```python
from build123d import *

# Parameters (mm, degrees)
BOSS_EXTRUDE1_DEPTH = 150
BOSS_EXTRUDE2_DEPTH = 150


with BuildPart() as part:
    # Sketch1 → Boss-Extrude1 (new body)
    with BuildSketch(Plane.XY):
        with BuildLine():
            Line((32.688132281, -32.688132281), (35.382209117, -35.382209117))
            ThreePointArc((35.382209117, -35.382209117), (0, -50.038), (-35.382209117, -35.382209117))
            Line((-35.382209117, -35.382209117), (-32.688132281, -32.688132281))
            ThreePointArc((-32.688132281, -32.688132281), (0, -46.228), (32.688132281, -32.688132281))
        make_face()
    extrude(amount=-BOSS_EXTRUDE1_DEPTH)

    # Sketch2 → Boss-Extrude2 (add)
    with BuildSketch(Plane.XY):
        with BuildLine():
            Line((-9.525, -36.775), (-28.011200599, -36.775))
            ThreePointArc((-28.011200599, -36.775), (-14.781631913, -43.801042704), (0, -46.228))
            Line((0, -46.228), (0, -45.609510869))
            Line((0, -45.609510869), (-4.445, -45.609510869))
            Line((-4.445, -45.609510869), (-4.445, -44.085510869))
            Line((-4.445, -44.085510869), (-12.622621116, -44.085510869))
            ThreePointArc((-12.622621116, -44.085510869), (-13.192135307, -43.731364187), (-13.126400487, -43.063947362))
            Line((-13.126400487, -43.063947362), (-9.525, -38.370510869))
            Line((-9.525, -38.370510869), (-9.525, -36.775))
        make_face()
        with BuildLine():
            Line((0, -45.609510869), (0, -46.228))
            ThreePointArc((0, -46.228), (14.781631913, -43.801042704), (28.011200599, -36.775))
            Line((28.011200599, -36.775), (9.525, -36.775))
            Line((9.525, -36.775), (9.525, -38.370510869))
            Line((9.525, -38.370510869), (13.126400487, -43.063947362))
            ThreePointArc((13.126400487, -43.063947362), (13.192135307, -43.731364187), (12.622621116, -44.085510869))
            Line((12.622621116, -44.085510869), (4.445, -44.085510869))
            Line((4.445, -44.085510869), (4.445, -45.609510869))
            Line((4.445, -45.609510869), (0, -45.609510869))
        make_face()
    extrude(amount=-BOSS_EXTRUDE2_DEPTH)


solid = part.part
```
Can you work these out from the model? Positions are in its coordinate system, mm. A direction names the side the tool comes from. Give positions to 0.01 mm unless a question says otherwise; leave off trailing zeros. Loops run counter-clockwise (first coordinate to the right, second up) from the corner with the lowest first, then second, coordinate; pieces in that order, holes last. Notation, with made-up numbers: M -13.5,71 L 12.5,71 A23 ccw 12.5,92 Z; hole C 27.5,76.25 d3. An arc over 180 degrees is marked long. Use CSV: the item, a comma, the result in double quotes. Start each with the question number.
1. If I drill on L1, parallel to X at y = -36, z = -101.5; L2, parallel to Y at x = -1, z = -116; L3, parallel to X at y = -40.25, z = -141, over which ranges is the centre line in solid material (lowest first)?
2. For P1, Ø0.8, axis at y = -45, z = -83, coming from the -X side; P2, Ø5, axis at x = -15.5, z = -130.5, coming from the +Y side (3 decimals); P3, Ø0.8, axis at y = -45, z = -70, coming from the +X side; P4, Ø8, axis at x = -19.5, y = -45, coming from the +Z side, each with a flat end and sliding along its axis, tell me the tip position at first contact or that it passes through.
3. Imagine slicing it at A-A, the plane z = -44. Write out the boundary of the cut face in (x, y) (3 decimals), plus the area to 3 significant figures.
4. If we mould it in two halves opening along Y, with no side actions, what happens to faces 1 (the face through (0, -45.61, -74)), 2 (the face through (9, -44.086, -74)), 3 (the face through (0.55, -50.035, -73.95))? For each: released by +Y, released by -Y, zero draft, split by the parting line, or undercut.
5. On a 3-axis mill with a long thin cutter (end or side, diameter ignored), from which of +Z, -Z, +X, -X, +Y, -Y can I reach the whole of each face in a straight line? I mean faces 4 (the face through (-30.45, -34.78, -73.95)), 5 (the face through (-8, -44.086, -74)), 6 (the face through (34, -34, -74)). Say none if no direction works.
Response values:
1,L1,"-34.75 to -29, 29 to 34.75"
1,L2,"-50.03 to -45.61"
1,L3,"-29.73 to -10.97, 10.97 to 29.73"
2,P1,"x = -22.69"
2,P2,"y = -36.775"
2,P3,"x = 22.69"
2,P4,"z = 0"
3,outline,"M -35.382,-35.382 A50.038 ccw 35.382,-35.382 L 32.688,-32.688 A46.228 cw 28.011,-36.775 L 9.525,-36.775 L 9.525,-38.371 L 13.126,-43.064 A0.635 cw 12.623,-44.086 L 4.445,-44.086 L 4.445,-45.61 L -4.445,-45.61 L -4.445,-44.086 L -12.623,-44.086 A0.635 cw -13.126,-43.064 L -9.525,-38.371 L -9.525,-36.775 L -28.011,-36.775 A46.228 cw -32.688,-32.688 Z"
3,area,"472 mm^2"
4,face 1,"released by +Y"
4,face 2,"undercut"
4,face 3,"released by -Y"
5,face 4,"+Z, -Z, +Y"
5,face 5,"+Z, -Z"
5,face 6,"+Z, -Z, +X, +Y"
